Input: part model. Units: mm. Frame: model coordinates. A direction names the side the tool comes from. Give positions to 0.01 mm unless a question says otherwise; leave off trailing zeros. Order: outer loops, then holes, each group sorted by start corner. A loop starts at its lowest first (then second) coordinate and runs counter-clockwise, first axis right, second up. Notation, with made-up numbers: (82, 55) - (86, 55) arc R32 ccw to (86, 84) - close; hole circle Ø3 at (13.5, -12). An arc over 180 degrees is marked (long way). Answer in a Markdown table with one row per item. Add a question column.
Autodesk Inventor part; units mm, degrees
ref_plane "YZ Plane" through (0, 0, 0) normal (1, 0, 0) x (0, 1, 0)
ref_plane "XZ Plane" through (0, 0, 0) normal (0, 1, 0) x (-1, 0, 0)
ref_plane "XY Plane" through (0, 0, 0) normal (0, 0, 1) x (1, 0, 0)
sketch "Sketch1" plane through (0, 0, 0) normal (0, 1, 0) x (-1, 0, 0)
  line L0 (8.0502, -54.6054) -> (-23.4458, -54.6054)
  line L1 (-23.4458, -54.6054) -> (-23.4458, 45.4706)
  line L2 (-23.4458, 45.4706) -> (8.0502, 45.4706)
  line L3 (8.0502, 45.4706) -> (8.0502, -54.6054)
  line L4 (10.5902, -57.1454) -> (-25.9858, -57.1454)
  line L5 (-25.9858, -57.1454) -> (-25.9858, 48.0106)
  line L6 (-25.9858, 48.0106) -> (10.5902, 48.0106)
  line L7 (10.5902, 48.0106) -> (10.5902, -57.1454)
  point P0 (0, 0)
  point P1 (-7.6978, -57.1454)
  dimension "d0" = 100.076
  dimension "d1" = 31.496
  dimension "d2" = 2.54
  dimension "d3" = 2.54
  dimension "d4" = 2.54
  dimension "d5" = 2.54
extrude "Extrusion1" add sketch "Sketch1" against normal blind 12.7508 contours L0 L1 L2 L3 | L4 L5 L6 L7
extrude "Extrusion2" cut sketch "Sketch1" against normal blind 10.2108 contours L0 L1 L2 L3
sketch "Sketch2" plane through (0, -10.2108, 0) normal (0, 1, 0) x (1, 0, 0)
  circle A0 centre (-5.0022, -42.4226) radius 1.143
  line L0 (-8.0502, -45.4706) -> (-8.0502, 54.6054)
  line L1 (23.4458, -45.4706) -> (-8.0502, -45.4706)
  arc A1 (-2.5892, -42.4226) -> (-5.0022, -40.0096) centre (-5.0022, -42.4226) ccw
  line L2 (-5.0022, -40.0096) -> (-8.0502, -40.0096)
  line L3 (-2.5892, -42.4226) -> (-2.5892, -45.4706)
  line L4 (23.4458, -45.4706) -> (-8.0502, -45.4706)
  line L5 (-8.0502, -45.4706) -> (-2.5892, -45.4706)
  line L6 (-8.0502, -40.0096) -> (-8.0502, -45.4706)
  line L7 (23.4458, 54.6054) -> (23.4458, -45.4706)
  line L8 (-8.0502, 54.6054) -> (23.4458, 54.6054)
  line L9 (-8.0502, 4.5674) -> (30.3732, 4.5674)
  line L10 (7.6978, -45.4706) -> (7.6978, 57.2864)
  circle A2 centre (20.3978, -42.4226) radius 1.143
  line L11 (23.4458, -45.4706) -> (23.4458, 54.6054)
  line L12 (-8.0502, -45.4706) -> (23.4458, -45.4706)
  arc A3 (20.3978, -40.0096) -> (17.9848, -42.4226) centre (20.3978, -42.4226) ccw
  line L13 (20.3978, -40.0096) -> (23.4458, -40.0096)
  line L14 (17.9848, -42.4226) -> (17.9848, -45.4706)
  line L15 (-8.0502, -45.4706) -> (23.4458, -45.4706)
  line L16 (23.4458, -40.0096) -> (23.4458, -45.4706)
  circle A4 centre (-5.0022, 51.5574) radius 1.143
  line L17 (23.4458, 54.6054) -> (-8.0502, 54.6054)
  arc A5 (-5.0022, 49.1444) -> (-2.5892, 51.5574) centre (-5.0022, 51.5574) ccw
  line L18 (-5.0022, 49.1444) -> (-8.0502, 49.1444)
  line L19 (-2.5892, 51.5574) -> (-2.5892, 54.6054)
  line L20 (23.4458, 54.6054) -> (-8.0502, 54.6054)
  line L21 (-8.0502, 54.6054) -> (-2.5892, 54.6054)
  line L22 (-8.0502, 49.1444) -> (-8.0502, 54.6054)
  circle A6 centre (20.3978, 51.5574) radius 1.143
  arc A7 (17.9848, 51.5574) -> (20.3978, 49.1444) centre (20.3978, 51.5574) ccw
  line L23 (17.9848, 51.5574) -> (17.9848, 54.6054)
  line L24 (-8.0502, 54.6054) -> (23.4458, 54.6054)
  line L25 (20.3978, 49.1444) -> (23.4458, 49.1444)
  line L26 (-8.0502, 54.6054) -> (23.4458, 54.6054)
  line L27 (23.4458, 49.1444) -> (23.4458, 54.6054)
  point P0 (0, 0)
  point P1 (7.6978, 54.6054)
  dimension "d10" = 2.286
  dimension "d11" = 3.048
  dimension "d12" = 3.048
  dimension "d13" = 4.826
extrude "Extrusion3" add sketch "Sketch2" along normal blind 8.636 contours L0 L2 A1 L3 L1 | L0 L8 L19 A5 L18 | L14 A3 L13 L7 L1 | L25 A7 L23 L8 L7
fillet "Fillet1" radius 1.27 8 edges at (7.6978, -12.7508, 48.0106) (25.9858, -6.3754, 48.0106) (25.9858, -12.7508, -4.5674) (25.9858, -6.3754, -57.1454) (-10.5902, -6.3754, 48.0106) (-10.5902, -12.7508, -4.5674) (-10.5902, -6.3754, -57.1454) (7.6978, -12.7508, -57.1454)
fillet "Fillet2" radius 1.27 16 edges at (-8.0502, -10.2108, -4.5674) (7.6978, -10.2108, -54.6054) (-6.5262, -10.2108, -49.1444) (-2.5892, -10.2108, -53.0814) (-3.296, -10.2108, -49.8511) (17.9848, -10.2108, -53.0814) (21.9218, -10.2108, -49.1444) (18.6915, -10.2108, -49.8511) (23.4458, -10.2108, -4.5674) (21.9218, -10.2108, 40.0096) (17.9848, -10.2108, 43.9466) (18.6915, -10.2108, 40.7164) (7.6978, -10.2108, 45.4706) (-2.5892, -10.2108, 43.9466) (-6.5262, -10.2108, 40.0096) (-3.296, -10.2108, 40.7164)
properties part number "CaseBottom"
Q1. Contact query for flat-ended pins moving along their axis: P1, Ø1.6, axis at x = 20, z = -52.5, coming from the +Y side; P2, Ø0.7, axis at x = 20, z = -52, coming from the +Y side. Output: stop coordinate, or through.
Q2. Section A-A, the plane y = -3.75. Return loops of the section in (x, z), then the cut area to 3 significant figures.
Q3. Section C-C, the plane z = 29. Return loops of the section in (x, y).
Q4. Pull-direction query (Z, two-part tool) for faces 1 (the flat face through (8, -6, 48.011)), 2 (the cylindrical face through (-3.31, -5.31, 40.7)), 3 (the flat face through (-10.59, -6, -4)); classes: +Z half, -Z half, draft (parallel to the pull), parting line (faces both ways), or undercut.
Q5. Line query: probe 1 along X at (y, z) = (-2.5, -40.5); probe 2 along Z at (x, y) = (12.5, -5.25); probe 3 along Z at (x, y) = (23, -8). Output: solid intervals per line, ascending.
Q6. Section B-B, the plane x = 7. Return loops of the section in (y, z), then the cut area to 3 significant figures.
Q7. Access query for faces 4 (the flat face through (25.986, -6, -5)), 5 (the flat face through (17.985, -5, 44)). Directions: +Z, -Z, +X, -X, +Y, -Y. A direction counts if a zero-diameter tool reaches every point of the face in a straight line with its end or side. Return the directions, or none.
Computed:
| question | item | result |
|---|---|---|
| 1 | P1 | stops at y = -1.57 |
| 1 | P2 | stops at y = -10.21 |
| 2 | outline | (-10.59, -55.88) arc R1.27 ccw to (-9.32, -57.15) - (24.72, -57.15) arc R1.27 ccw to (25.99, -55.88) - (25.99, 46.74) arc R1.27 ccw to (24.72, 48.01) - (-9.32, 48.01) arc R1.27 ccw to (-10.59, 46.74) - close; hole (-8.05, -49.14) - (-5, -49.14) arc R2.41 cw to (-2.59, -51.56) - (-2.59, -54.61) - (17.98, -54.61) - (17.98, -51.56) arc R2.41 cw to (20.4, -49.14) - (23.45, -49.14) - (23.45, 40.01) - (20.4, 40.01) arc R2.41 cw to (17.98, 42.42) - (17.98, 45.47) - (-2.59, 45.47) - (-2.59, 42.42) arc R2.41 cw to (-5, 40.01) - (-8.05, 40.01) - close; hole circle Ø2.29 at (-5, -51.56); hole circle Ø2.29 at (-5, 42.42); hole circle Ø2.29 at (20.4, -51.56); hole circle Ø2.29 at (20.4, 42.42) |
| 2 | area | 791 mm^2 |
| 3 | outline | (-10.59, -11.48) arc R1.27 ccw to (-9.32, -12.75) - (24.72, -12.75) arc R1.27 ccw to (25.99, -11.48) - (25.99, 0) - (23.45, 0) - (23.45, -8.94) arc R1.27 cw to (22.18, -10.21) - (-6.78, -10.21) arc R1.27 cw to (-8.05, -8.94) - (-8.05, 0) - (-10.59, 0) - close |
| 4 | face 1 | +Z half |
| 4 | face 2 | undercut |
| 4 | face 3 | draft |
| 5 | probe 1 | x = -10.59 to -8.05, 23.45 to 25.99 |
| 5 | probe 2 | z = -57.15 to -54.61, 45.47 to 48.01 |
| 5 | probe 3 | z = -57.15 to -49.14, 40.01 to 48.01 |
| 6 | outline | (-12.75, -55.88) arc R1.27 ccw to (-11.48, -57.15) - (0, -57.15) - (0, -54.61) - (-8.94, -54.61) arc R1.27 cw to (-10.21, -53.34) - (-10.21, 44.2) arc R1.27 cw to (-8.94, 45.47) - (0, 45.47) - (0, 48.01) - (-11.48, 48.01) arc R1.27 ccw to (-12.75, 46.74) - close |
| 6 | area | 319 mm^2 |
| 7 | face 4 | +Z, -Z, +X, +Y, -Y |
| 7 | face 5 | +Y |
